Source: CAD feature listing. Evaluate the final solid. Frame: model axes, mm. A direction names the side the tool comes from. Give positions to 0.01 mm unless a question says otherwise; leave off trailing zeros. Order: outer loops, then holes, each group sorted by start corner. A loop starts at its lowest first (then second) coordinate and runs counter-clockwise, first axis right, second up. Notation, with made-up numbers: M 38,47 L 92,47 A15 cw 92,65 Z; hole C 11.5,46.5 d1. An arc over 180 degrees is marked long. Return JSON: item names as keys, results as strings.
from build123d import *

# Parameters (mm, degrees)
BOSS_EXTRUDE1_DEPTH         = 76.2
BOSS_EXTRUDE2_DEPTH         = 381
F_1_4_20_TAPPED_HOLE3_D     = 5.1054
F_1_4_20_TAPPED_HOLE3_DEPTH = 19.05
F_1_4_20_TAPPED_HOLE3_TIP   = 1.533816902
F_1_4_20_TAPPED_HOLE2_D     = 5.1054
F_1_4_20_TAPPED_HOLE2_DEPTH = 19.05
F_1_4_20_TAPPED_HOLE2_TIP   = 1.533816902
F_3_8_16_TAPPED_HOLE1_D     = 7.9375
F_3_8_16_TAPPED_HOLE1_DEPTH = 26.924
F_3_8_16_TAPPED_HOLE1_TIP   = 2.384665582
F_1_4_20_TAPPED_HOLE1_D     = 5.1054
F_1_4_20_TAPPED_HOLE1_DEPTH = 17.4625
F_1_4_20_TAPPED_HOLE1_TIP   = 1.533816902
CHAMFER1_SIZE               = 20.492049699
CHAMFER1_SIZE2              = 2.998111049


with BuildPart() as part:
    # Sketch1 → Boss-Extrude1 (new body)
    with BuildSketch(Plane(origin=(0, 0, -76.2), x_dir=(-1, 0, 0), z_dir=(0, 0, -1))):
        with BuildLine():
            Line((0, 0), (0, 25.4))
            Line((0, 25.4), (-101.6, 36.5125))
            Line((-101.6, 36.5125), (-142.723305624, 36.5125))
            Line((-142.723305624, 36.5125), (-127, 19.05))
            Line((-127, 19.05), (-158.75, 19.05))
            ThreePointArc((-158.75, 19.05), (-159.214967985, 17.927467985), (-160.3375, 17.4625))
            Line((-160.3375, 17.4625), (-220.6625, 17.4625))
            ThreePointArc((-220.6625, 17.4625), (-221.785032015, 17.927467985), (-222.25, 19.05))
            Line((-222.25, 19.05), (-266.7, 19.05))
            Line((-266.7, 19.05), (-284.429433488, 38.740530712))
            Line((-284.429433488, 38.740530712), (-406.4, 25.4))
            Line((-406.4, 25.4), (-406.4, 0))
            Line((-406.4, 0), (0, 0))
        make_face()
    extrude(amount=-BOSS_EXTRUDE1_DEPTH)

    # Sketch2 → Boss-Extrude2 (add)
    with BuildSketch(Plane(origin=(0, 0, 0), x_dir=(0, -1, 0), z_dir=(-1, 0, 0))):
        Polygon((0, -25.4), (0, -50.8), (9.525, -50.8), (9.525, -60.325), (19.05, -60.325), (19.05, -15.875), (9.525, -15.875), (9.525, -25.4), align=None)
    extrude(amount=-BOSS_EXTRUDE2_DEPTH)

    # 1/4-20 Tapped Hole3
    with Locations(Plane(origin=(0, 0, 0), x_dir=(-1, 0, 0), z_dir=(0, -1, 0))):
        with Locations((-393.7, 65.0875), (-393.7, 11.1125)):
            Hole(F_1_4_20_TAPPED_HOLE3_D / 2, depth=F_1_4_20_TAPPED_HOLE3_DEPTH)
            with Locations((0, 0, -(F_1_4_20_TAPPED_HOLE3_DEPTH + F_1_4_20_TAPPED_HOLE3_TIP / 2))):  # 118° drill point
                Cone(0, F_1_4_20_TAPPED_HOLE3_D / 2, F_1_4_20_TAPPED_HOLE3_TIP, mode=Mode.SUBTRACT)

    # 1/4-20 Tapped Hole2
    with Locations(Plane(origin=(0, 0, -76.2), x_dir=(-1, 0, 0), z_dir=(0, 0, -1))):
        with Locations((-139.7, 9.525), (-241.3, 9.525)):
            Hole(F_1_4_20_TAPPED_HOLE2_D / 2, depth=F_1_4_20_TAPPED_HOLE2_DEPTH)
            with Locations((0, 0, -(F_1_4_20_TAPPED_HOLE2_DEPTH + F_1_4_20_TAPPED_HOLE2_TIP / 2))):  # 118° drill point
                Cone(0, F_1_4_20_TAPPED_HOLE2_D / 2, F_1_4_20_TAPPED_HOLE2_TIP, mode=Mode.SUBTRACT)

    # 3/8-16 Tapped Hole1
    with Locations(Plane(origin=(0, 19.05, 0), x_dir=(1, 0, 0), z_dir=(0, 1, 0))):
        with Locations((260.35, 38.1)):
            Hole(F_3_8_16_TAPPED_HOLE1_D / 2, depth=F_3_8_16_TAPPED_HOLE1_DEPTH)
            with Locations((0, 0, -(F_3_8_16_TAPPED_HOLE1_DEPTH + F_3_8_16_TAPPED_HOLE1_TIP / 2))):  # 118° drill point
                Cone(0, F_3_8_16_TAPPED_HOLE1_D / 2, F_3_8_16_TAPPED_HOLE1_TIP, mode=Mode.SUBTRACT)

    # 1/4-20 Tapped Hole1
    with Locations(Plane(origin=(0, 19.05, 0), x_dir=(1, 0, 0), z_dir=(0, 1, 0))):
        with Locations((260.35, 12.7), (260.35, 63.5)):
            Hole(F_1_4_20_TAPPED_HOLE1_D / 2, depth=F_1_4_20_TAPPED_HOLE1_DEPTH)
            with Locations((0, 0, -(F_1_4_20_TAPPED_HOLE1_DEPTH + F_1_4_20_TAPPED_HOLE1_TIP / 2))):  # 118° drill point
                Cone(0, F_1_4_20_TAPPED_HOLE1_D / 2, F_1_4_20_TAPPED_HOLE1_TIP, mode=Mode.SUBTRACT)

    # Chamfer1
    chamfer1_edges = [part.edges().sort_by_distance(p)[0] for p in [
        (284.429433488, 38.740530712, -38.1),
    ]]
    chamfer1_side = [part.faces().sort_by_distance(p)[0] for p in [
        (345.414716744, 32.070265356, -38.1),
    ]]
    chamfer(chamfer1_edges, length=CHAMFER1_SIZE, length2=CHAMFER1_SIZE2, reference=chamfer1_side[0])


solid = part.part
1. First-contact query: pin 1 (3 mm diameter, centred on x = 393.7, z = -11.11, fed in from +Y); pin 2 (18 mm diameter, centred on x = 199, z = -52, fed in from +Y); pin 3 (3 mm diameter, centred on x = 97, y = -14.5, fed in from -Z) (3 decimals). Flat tips, straight axial feed; report the tip coordinate or a pass-through.
Evaluation:
{"pin 1": "stops at y = 26.95", "pin 2": "stops at y = 17.46", "pin 3": "stops at z = -60.325"}
2. Set-up query: faces 1 (the face through (188, -5, -50.8)), 2 (the face through (190, 17.462, -39)), 3 (the face through (188, -14, -15.875)), 4 (the face through (188, -14, -60.325)). Return all of +Z, -Z, +X, -X, +Y, -Y with unobstructed straight access to the full face (end or side cutting, diameter ignored); none if empty.
Evaluation:
{"face 1": "-Z, +X, -X", "face 2": "+Z, -Z, +Y", "face 3": "+Z, +X, -X, -Y", "face 4": "-Z, +X, -X, -Y"}
3. Draft query along X for faces 5 (the face through (244, 19.05, -39)), 6 (the face through (381, -12, -38)), 7 (the face through (261.007, -9.845, -38.307)), 8 (the face through (188, -9.525, -21)). Return one class per face: pulls with the +X half, pulls with the -X half, needs draft (parallel to the pull), parting line crosses it, or undercut.
Evaluation:
{"face 5": "undercut", "face 6": "pulls with the +X half", "face 7": "undercut", "face 8": "needs draft"}
4. Section query B-B (x = 28.5). Return loops of the section in (y, z) (3 decimals).
Evaluation:
{"outline": "M -19.05,-60.325 L -9.525,-60.325 L -9.525,-50.8 L 0,-50.8 L 0,-76.2 L 28.517,-76.2 L 28.517,0 L 0,0 L 0,-25.4 L -9.525,-25.4 L -9.525,-15.875 L -19.05,-15.875 Z"}
5. Ray query, probe 1 along Z at (x, y) = (260.35, 9.5); probe 2 along Z at (x, y) = (393.7, 15); probe 3 along X at (y, z) = (11, -62). Return the intervals inside material, ascending.
Evaluation:
{"probe 1": "z = -76.2 to -66.05, -60.95 to -42.07, -34.13 to -15.25, -10.15 to 0", "probe 2": "z = -76.2 to -67.64, -62.53 to -13.67, -8.56 to 0", "probe 3": "x = 0 to 137.62, 141.78 to 239.22, 243.38 to 258.28, 262.42 to 406.4"}
